Verification items for the finished model (mm, model axes). Face numbers are marked on the shaded views. A direction names the side the tool comes from. Round coordinates to 2 decimals unless told otherwise and drop trailing zeros. Write each loop counter-clockwise with the first axis right and the second up, starting at its lowest first coordinate (ties: lowest second). Pieces come first, ordered by that corner, then holes. Notation, with made-up numbers: (-15.5, -8) -> (28.5, -8) arc R21 cw to (28.5, -3) -> close; hole circle Ø6 at (53.25, -32). An arc over 180 degrees is marked (long way). Use CSV: the item, a comma, the result in double quotes.
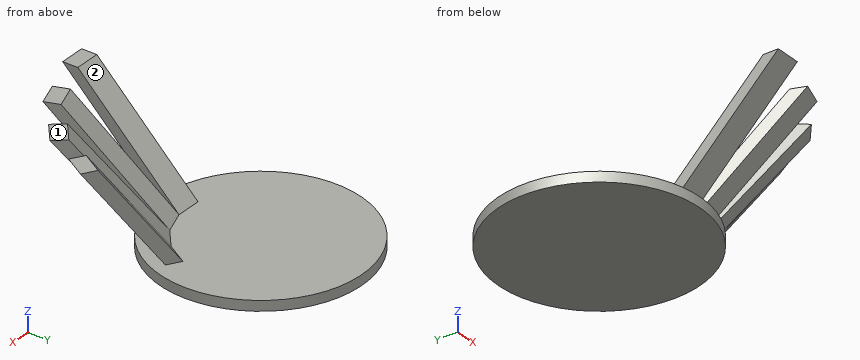
```python
from build123d import *

# Parameters (mm, degrees)
F3_DEPTH  = 2.5
F4_R      = 20
F5_DEPTH  = 2
F6_DEPTH  = 2.5
F9_DEPTH  = 2.5
F12_DEPTH = 2.5


with BuildPart() as f3:
    # F0 (on Right) → F3 (new body, symmetric)
    with BuildSketch(Plane.YZ):
        Polygon((-3, 0), (0, 0), (-20, 20), (-23, 20), align=None)
    extrude(amount=F3_DEPTH, both=True)

    # F4 (on Top) → F5 (join)
    with BuildSketch(Plane.XY):
        with Locations((0, 14.28)):
            Circle(F4_R)
    extrude(amount=-F5_DEPTH)

    # F2 (on line) → F6 (join, symmetric)
    with BuildSketch(Plane(origin=(4.5822124443, 1.6316524569, 0), x_dir=(0.3354515698, -0.9420574528, 0), z_dir=(-0.9420574528, -0.3354515698, 0))):
        Polygon((18.8401669346, 20), (0.8401669346, 0), (3.8401669346, 0), (21.8401669346, 20), align=None)
    extrude(amount=F6_DEPTH, both=True)

    # F8 (on line) → F9 (join, symmetric)
    with BuildSketch(Plane(origin=(7.1019205596, 5.7921850717, 0), x_dir=(0.6320293027, -0.7749444887, 0), z_dir=(-0.7749444887, -0.6320293027, 0))):
        Polygon((19.4633049138, 20), (3.2633049138, 0), (6.2633049138, 0), (22.4633049138, 20), align=None)
    extrude(amount=F9_DEPTH, both=True)

    # F11 (on line) → F12 (join, symmetric)
    with BuildSketch(Plane(origin=(6.4249759494, 10.6088962546, 0), x_dir=(0.8553642602, -0.5180270094, 0), z_dir=(-0.5180270094, -0.8553642602, 0))):
        Polygon((21.4886083641, 20), (6.9886083641, 0), (9.9886083641, 0), (24.4886083641, 20), align=None)
    extrude(amount=F12_DEPTH, both=True)


solid = f3.part
```
Q1. Material ranges on L1, parallel to Z at x = 14, y = 1.5; L2, parallel to X at y = 3, z = 14.25; L3, parallel to Y at x = 17, z = 10.75, recorded low to high.
Filled in:
L1,"-2 to 0"
L2,"22.07 to 23.81"
L3,"-5.45 to -2.39"
Q2. Access from +Z, -Z, +X, -X, +Y, -Y to the whole of each face (thin tool, end or side, straight path). Record for the marked faces 1 and 2.
Filled in:
face 1,"+Z, +X, -X, +Y, -Y"
face 2,"+Z, -X, +Y"
Q3. Section check C-C (y = 14.28). Record the cut outline in (x, z), plus the area to 3 significant figures.
Filled in:
outline,"(-20, -2) -> (20, -2) -> (20, 0) -> (-20, 0) -> close"
area,"80.0 mm²"
Q4. Go/stop test with flat-tipped pins: P1, Ø3, axis at x = 11, z = 13.5, coming from the +Y side; P2, Ø6, axis at x = 10.5, z = 17.5, coming from the -Y side; P3, Ø10, axis at x = -9, z = 1, coming from the +Y side (3 decimals). Record where each tip stops, or that it passes through.
Filled in:
P1,"y = -8.5"
P2,"y = -19.78"
P3,"y = 33.855"
Q5. Section check B-B (x = 0). Record the cut outline in (y, z).
Filled in:
outline,"(-23, 20) -> (-3, 0) -> (-5.72, 0) -> (-5.72, -2) -> (34.28, -2) -> (34.28, 0) -> (0, 0) -> (-20, 20) -> close"
Q6. Section check A-A (z = 6). Record the cut outline in (x, y).
Filled in:
outline,"(-2.5, -9) -> (2.5, -9) -> (2.5, -6) -> (-2.5, -6) -> close; (4.32, -5.09) -> (5.33, -7.91) -> (10.04, -6.23) -> (9.03, -3.41) -> close; (10.3, -2.08) -> (12.19, -4.41) -> (16.07, -1.25) -> (14.17, 1.08) -> close; (14.83, 2.6) -> (17.39, 1.04) -> (19.98, 5.32) -> (17.42, 6.87) -> close"
